Model file for the job. Use its own axes, mm. A direction names the side the tool comes from. Round coordinates to 2 decimals unless told otherwise and drop trailing zeros. Order: outer loops, then holes, each group sorted by start corner. A loop starts at its lowest first (then second) coordinate and runs counter-clockwise, first axis right, second up. Notation, with made-up numbers: (-27.5, 55.5) -> (12.5, 55.5) arc R22 ccw to (12.5, 67.5) -> close; hole circle Ø3 at (62.25, -30). An arc over 180 degrees is marked (long way). Answer as CSV lines item,"result".
```python
from build123d import *

# Parameters (mm, degrees)
DODANIE_WYCI_GNI_CIE1_DEPTH      = 30
DODANIE_WYCI_GNI_CIE1_DEPTH_BACK = 30
WYTNIJ_WYCI_GNI_CIE1_DEPTH       = 232.526456676
WYTNIJ_WYCI_GNI_CIE1_DEPTH_BACK  = 232.526456676
SZKIC2_W                         = 55
SZKIC2_H                         = 107.496477766
SZKIC3_W                         = 55
SZKIC3_H                         = 40
WYTNIJ_WYCI_GNI_CIE3_DEPTH       = 232.526456676
SZKIC4_W                         = 40
SZKIC4_H                         = 20
DODANIE_WYCI_GNI_CIE2_DEPTH      = 20
SZKIC5_W                         = 17.5
SZKIC5_H                         = 17.5
WYTNIJ_WYCI_GNI_CIE4_DEPTH       = 262.571382555
SZKIC6_R                         = 4
DODANIE_WYCI_GNI_CIE3_DEPTH      = 1
WYTNIJ_WYCI_GNI_CIE5_DEPTH       = 237.615194231
SZKIC8_R                         = 5
SZKIC8_R_2                       = 8
SZKIC8_R_3                       = 10
WYTNIJ_WYCI_GNI_CIE6_DEPTH       = 244.114171


with BuildPart() as part:
    # Szkic1 → Dodanie-wyci_gni_cie1 (new, two sides: drawn at the far end of the back side and taken through both)
    with BuildSketch(Plane(origin=(0, 0, 0), x_dir=(0, 0, -1), z_dir=(1, 0, 0)).offset(-DODANIE_WYCI_GNI_CIE1_DEPTH_BACK)):
        with BuildLine():
            Line((0, 0), (181.505583399, 0))
            ThreePointArc((181.505583399, 0), (201.334480627, 17.389476156), (186.681964301, 39.318516526))
            Line((186.681964301, 39.318516526), (32.133832095, 80.729563742))
            ThreePointArc((32.133832095, 80.729563742), (27.839163279, 82.875338226), (24.730497196, 86.533852072))
            Line((24.730497196, 86.533852072), (17.525057128, 99.637031321))
            ThreePointArc((17.525057128, 99.637031321), (0, 110), (-17.525057128, 99.637031321))
            Line((-17.525057128, 99.637031321), (-41.617635429, 55.824388502))
            Line((-41.617635429, 55.824388502), (-76.972974488, 20.469049442))
            ThreePointArc((-76.972974488, 20.469049442), (-79.572186332, 7.401929091), (-68.494416601, 0))
            Line((-68.494416601, 0), (0, 0))
        make_face()
    extrude(amount=DODANIE_WYCI_GNI_CIE1_DEPTH + DODANIE_WYCI_GNI_CIE1_DEPTH_BACK)

    # Szkic2 → Wytnij-wyci_gni_cie1 (cut, two sides: drawn at the far end of the back side and taken through both)
    with BuildSketch(Plane.XY.offset(-WYTNIJ_WYCI_GNI_CIE1_DEPTH_BACK)):
        with Locations((0, 56.251761117)):
            Rectangle(SZKIC2_W, SZKIC2_H)
    extrude(amount=WYTNIJ_WYCI_GNI_CIE1_DEPTH + WYTNIJ_WYCI_GNI_CIE1_DEPTH_BACK, mode=Mode.SUBTRACT)

    # Szkic3 → Wytnij-wyci_gni_cie3 (cut, through all)
    with BuildSketch(Plane(origin=(0, 0, 0), x_dir=(1, 0, 0), z_dir=(0, 1, 0))):
        with Locations((0, 171.194405091)):
            Rectangle(SZKIC3_W, SZKIC3_H)
    extrude(amount=WYTNIJ_WYCI_GNI_CIE3_DEPTH, mode=Mode.SUBTRACT)

    # Szkic4 → Dodanie-wyci_gni_cie2 (add)
    with BuildSketch(Plane(origin=(30, 0, 0), x_dir=(0, 0, -1), z_dir=(1, 0, 0))):
        with Locations((-48.494416601, 4)):
            Rectangle(SZKIC4_W, SZKIC4_H)
        with Locations((131.505583399, 4)):
            Rectangle(SZKIC4_W, SZKIC4_H)
    dodanie_wyci_gni_cie2 = extrude(amount=DODANIE_WYCI_GNI_CIE2_DEPTH)

    # Szkic5 → Wytnij-wyci_gni_cie4 (cut, through all)
    with BuildSketch(Plane(origin=(0, 0, -151.505583399), x_dir=(-1, 0, 0), z_dir=(0, 0, -1))):
        with Locations((-41.25, 5.25)):
            Rectangle(SZKIC5_W, SZKIC5_H)
    wytnij_wyci_gni_cie4 = extrude(amount=-WYTNIJ_WYCI_GNI_CIE4_DEPTH, mode=Mode.SUBTRACT)

    # Szkic6 → Dodanie-wyci_gni_cie3 (add)
    with BuildSketch(Plane(origin=(32.5, 0, 0), x_dir=(0, 0, -1), z_dir=(1, 0, 0))):
        with Locations(Location((-48.494416601, 7, 0), (0, 0, 180))):
            Circle(SZKIC6_R)
        with Locations(Location((131.505583399, 7, 0), (0, 0, 180))):
            Circle(SZKIC6_R)
    dodanie_wyci_gni_cie3 = extrude(amount=DODANIE_WYCI_GNI_CIE3_DEPTH)

    # Lustro2: Dodanie-wyci_gni_cie2, Wytnij-wyci_gni_cie4, Dodanie-wyci_gni_cie3 across plane
    add(dodanie_wyci_gni_cie2.mirror(Plane(origin=(0, 0, 0), x_dir=(0, 0, 1), z_dir=(1, 0, 0))))
    add(wytnij_wyci_gni_cie4.mirror(Plane(origin=(0, 0, 0), x_dir=(0, 0, 1), z_dir=(1, 0, 0))), mode=Mode.SUBTRACT)
    add(dodanie_wyci_gni_cie3.mirror(Plane(origin=(0, 0, 0), x_dir=(0, 0, 1), z_dir=(1, 0, 0))))

    # Szkic7 → Wytnij-wyci_gni_cie5 (cut, through all)
    with BuildSketch(Plane(origin=(0, -3.5, 0), x_dir=(1, 0, 0), z_dir=(0, 1, 0))):
        with BuildLine():
            Line((-37.25, 145.505583399), (-37.25, 117.505583399))
            ThreePointArc((-37.25, 117.505583399), (-41.25, 113.505583399), (-45.25, 117.505583399))
            Line((-45.25, 117.505583399), (-45.25, 145.505583399))
            ThreePointArc((-45.25, 145.505583399), (-41.25, 149.505583399), (-37.25, 145.505583399))
        make_face()
        with BuildLine():
            Line((-37.25, -34.494416601), (-37.25, -62.494416601))
            ThreePointArc((-37.25, -62.494416601), (-41.25, -66.494416601), (-45.25, -62.494416601))
            Line((-45.25, -62.494416601), (-45.25, -34.494416601))
            ThreePointArc((-45.25, -34.494416601), (-41.25, -30.494416601), (-37.25, -34.494416601))
        make_face()
    wytnij_wyci_gni_cie5 = extrude(amount=-WYTNIJ_WYCI_GNI_CIE5_DEPTH, mode=Mode.SUBTRACT)

    # Lustro3: Wytnij-wyci_gni_cie5 across plane
    add(wytnij_wyci_gni_cie5.mirror(Plane(origin=(0, 0, 0), x_dir=(0, 0, 1), z_dir=(1, 0, 0))), mode=Mode.SUBTRACT)

    # Szkic8 → Wytnij-wyci_gni_cie6 (cut, through all)
    with BuildSketch(Plane(origin=(30, 0, 0), x_dir=(0, 0, -1), z_dir=(1, 0, 0))):
        with Locations((0, 98)):
            Circle(SZKIC8_R)
        with Locations((-51.634860528, 31.718842875)):
            Circle(SZKIC8_R)
        with Locations((0, 80)):
            Circle(SZKIC8_R_2)
        with Locations((0, 58)):
            Circle(SZKIC8_R_3)
        with Locations((181.505583399, 20)):
            Circle(SZKIC8_R_2)
    extrude(amount=-WYTNIJ_WYCI_GNI_CIE6_DEPTH, mode=Mode.SUBTRACT)


solid = part.part
```
Q1. Saw through at A-A (z = 0). State how many separate pieces and enclosed holes the cut face has, plus the area to 3 significant figures.
Checks:
separate pieces,"7"
enclosed holes,"0"
area,"458 mm²"
Q2. Saw through at B-B (x = 41.25). Write the cut outline in (y, z).
Checks:
outline,"(-6, -151.51) -> (-3.5, -151.51) -> (-3.5, -149.51) -> (-6, -149.51) -> close; (-6, -113.51) -> (-3.5, -113.51) -> (-3.5, -111.51) -> (-6, -111.51) -> close; (-6, 28.49) -> (-3.5, 28.49) -> (-3.5, 30.49) -> (-6, 30.49) -> close; (-6, 66.49) -> (-3.5, 66.49) -> (-3.5, 68.49) -> (-6, 68.49) -> close"
Q3. Tool access for faces 1 (the flat face through (-36, -4, -111.506)), 2 (the flat face through (36, -4, 28.494)), 3 (the flat face through (-33.5, 7, 48)), 4 (the flat face through (0, 2.504, -39)): list every direction of +Z, -Z, +X, -X, +Y, -Y with a clear straight run to the whole face (end or side of a thin tool).
Checks:
face 1,"-X, +Y, -Y"
face 2,"+X, +Y, -Y"
face 3,"+Z, -Z, -X, +Y"
face 4,"+Z, -Z, +Y"
Q4. Mould opens along X. For faces 5 (the flat face through (-28.77, 92.99, -21.18)), 6 (the flat face through (33.5, 7, -132)), 7 (the flat face through (27.5, 30, -59)) say: +X half, -X half, draft (parallel to the pull), parting line (faces both ways), or undercut.
Checks:
face 5,"draft"
face 6,"+X half"
face 7,"undercut"
Q5. Saw through at D-D (x = 4.5). Write the cut outline in (y, z), plus the area to 3 significant figures.
Checks:
outline,"(0, -151.19) -> (2.5, -151.19) -> (2.5, 75.83) arc R11.99 ccw to (0, 68.49) -> close"
area,"563 mm²"
Q6. Wall check: L1, parallel to Y at x = -29.5, z = 0; L2, parallel to X at y = 17, z = -10; L3, parallel to X at y = 1, z = 54. Give the ranges that are in metal, low to high. Write a range as [from, to].
Checks:
L1,"[0, 48], [68, 72], [88, 93], [103, 110]"
L2,"[-30, -27.5], [27.5, 30]"
L3,"[-32.5, 32.5]"
Q7. Flat gauge pins, fed straight in: pin 1 (0.8 mm diameter, centred on x = 31.5, z = 40.5, fed in from +Y); pin 2 (6.5 mm diameter, centred on y = 6.5, z = 48.5, fed in from +X); pin 3 (1 mm diameter, centred on y = 52, z = -93.5, fed in from +X); pin 4 (14.5 mm diameter, centred on y = 20, z = -181.51, fed in from -X). Where does each tip first touch, or does it go through?
Checks:
pin 1,"y = 14"
pin 2,"x = 33.5"
pin 3,"x = 30"
pin 4,"through"
Q8. Saw through at C-C (z = -41). Write the cut outline in (x, y).
Checks:
outline,"(-30, 0) -> (30, 0) -> (30, 78.35) -> (27.5, 78.35) -> (27.5, 2.5) -> (-27.5, 2.5) -> (-27.5, 78.35) -> (-30, 78.35) -> close"
